Here's how the part is built. I have some questions about the finished solid (model axes, mm). Face numbers are marked on the shaded views. A direction names the side the tool comes from. Coordinates: 2 decimals unless noted, no trailing zeros. Write each loop counter-clockwise with the first axis right and the second up, starting at its lowest first coordinate (ties: lowest second). Pieces come first, ordered by that corner, then holes. Notation, with made-up numbers: M 71.25,26 L 123.25,26 A23 cw 123.25,55 Z; hole C 28.25,83 d7. An arc over 180 degrees is marked long. Write each question's results on one line, items separated by ' | '. Start each with the question number.
from build123d import *

# Parameters (mm, degrees)
SKETCH1_W           = 20
SKETCH1_H           = 24
BOSS_EXTRUDE1_DEPTH = 30
CUT_EXTRUDE1_DEPTH  = 21
SKETCH3_W           = 16
SKETCH3_H           = 19
CUT_EXTRUDE2_DEPTH  = 27
SKETCH4_W           = 14
SKETCH4_H           = 14
BOSS_EXTRUDE2_DEPTH = 12
SKETCH5_R           = 1.6
CUT_EXTRUDE3_DEPTH  = 31
SKETCH6_R           = 2
CUT_EXTRUDE4_DEPTH  = 4


with BuildPart() as part:
    # Sketch1 → Boss-Extrude1 (new body)
    with BuildSketch(Plane.XY):
        Rectangle(SKETCH1_W, SKETCH1_H)
    extrude(amount=BOSS_EXTRUDE1_DEPTH)

    # Sketch2 → Cut-Extrude1 (cut, through all)
    with BuildSketch(Plane(origin=(10, 0, 0), x_dir=(0, 0, -1), z_dir=(1, 0, 0))):
        Polygon((0, -12), (-30, 9), (-30, -12), align=None)
    extrude(amount=-CUT_EXTRUDE1_DEPTH, mode=Mode.SUBTRACT)

    # Sketch3 → Cut-Extrude2 (cut)
    with BuildSketch(Plane.XY.offset(30)):
        with Locations((0, -0.5)):
            Rectangle(SKETCH3_W, SKETCH3_H)
    extrude(amount=-CUT_EXTRUDE2_DEPTH, mode=Mode.SUBTRACT)

    # Sketch4 → Boss-Extrude2 (add)
    with BuildSketch(Plane.XY.offset(3)):
        Rectangle(SKETCH4_W, SKETCH4_H)
    extrude(amount=BOSS_EXTRUDE2_DEPTH)

    # Sketch5 → Cut-Extrude3 (cut, through all)
    with BuildSketch(Plane(origin=(0, 0, 0), x_dir=(-1, 0, 0), z_dir=(0, 0, -1))):
        Circle(SKETCH5_R)
    extrude(amount=-CUT_EXTRUDE3_DEPTH, mode=Mode.SUBTRACT)

    # Sketch6 → Cut-Extrude4 (cut, through all)
    with BuildSketch(Plane.XZ.offset(-9)):
        with Locations((0, 22)):
            Circle(SKETCH6_R)
    extrude(amount=-CUT_EXTRUDE4_DEPTH, mode=Mode.SUBTRACT)


solid = part.part
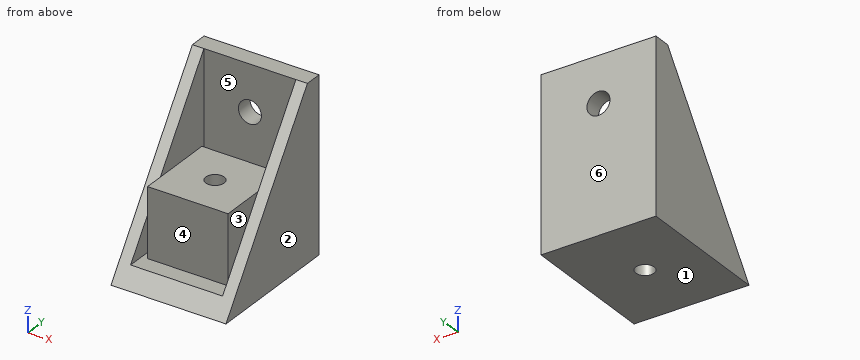
1) I want a section at C-C, the plane y = 0. Write out the boundary of the cut face in (x, z).
2) Please list where these lines run through material, in increasing order: line 1 (Y direction, x = 0, z = 5.75); line 2 (Y direction, x = -4.75, z = 10.5); line 3 (Z direction, x = 0, y = 10.6). Write a range as [from, to].
3) For the marked faces 4, 5 and 6, which set-ups out of +Z, -Z, +X, -X, +Y, -Y let a thin tool reach every point of the face, with its end or its side?
4) We'd pull the mould along X, two halves only. Please class the marked faces 1, 2 and 3: pulls with the +X half, pulls with the -X half, needs draft (parallel to the pull), parting line crosses it, or undercut.
5) I want a section at D-D, the plane y = 3.75. Write out the boundary of the cut face in (x, z), then the cut area to 3 significant figures.
6) I want a section at B-B, the plane z = 22. Write out the boundary of the cut face in (x, y).
7) For pin 1 Ø5 at (x, y) = (0, 0) entering from +Z; pin 2 Ø9.5 at (x, z) = (-0.5, 12) entering from -Y; pin 3 Ø3 at (x, z) = (7, 22.5) entering from -Y, each with a flat end and sliding along its axis, tell me the tip position at first contact or that it passes through.
8) I want a section at A-A, the plane x = 0. Write out the boundary of the cut face in (y, z).
Output:
1) outline: M -10,0 L -1.6,0 L -1.6,15 L -7,15 L -7,3 L -8,3 L -8,17.14 L -10,17.14 Z; M 1.6,0 L 10,0 L 10,17.14 L 8,17.14 L 8,3 L 7,3 L 7,15 L 1.6,15 Z
2) line 1: y = [-7, -1.6], [1.6, 7], [9, 12] | line 2: y = [-7, 7], [9, 12] | line 3: z = [0, 20], [24, 30]
3) face 4: +Z, -Y | face 5: +Z | face 6: +Z, -Z, +X, -X, +Y
4) face 1: needs draft | face 2: pulls with the +X half | face 3: undercut
5) outline: M -10,0 L 10,0 L 10,22.5 L 8,22.5 L 8,3 L 7,3 L 7,15 L -7,15 L -7,3 L -8,3 L -8,22.5 L -10,22.5 Z | area: 306 mm2
6) outline: M -10,3.4 L -8,3.4 L -8,9 L -2,9 L -2,12 L -10,12 Z; M 2,9 L 8,9 L 8,3.4 L 10,3.4 L 10,12 L 2,12 Z
7) pin 1: stops at z = 15 | pin 2: stops at y = -7 | pin 3: stops at y = 2.97
8) outline: M -12,0 L -1.6,0 L -1.6,15 L -7,15 L -7,3 L -9.9,3 Z; M 1.6,0 L 12,0 L 12,20 L 9,20 L 9,3 L 7,3 L 7,15 L 1.6,15 Z; M 9,24 L 12,24 L 12,30 L 9,30 Z
